Check sheet for the drawn part. Datum: minimum x, y, z corner. Units: mm. A direction names the side the tool comes from. Give positions to 0.01 mm unless a question says otherwise; leave off trailing zeros. Loops run counter-clockwise (first coordinate to the right, second up) from the corner with the lowest first, then second, coordinate; pieces in that order, holes last. Notation, with made-up numbers: (33.5, 71.5) - (59.5, 71.5) arc R22 ccw to (59.5, 106.5) - close; hole circle Ø2 at (23, 10.25). An arc over 180 degrees is marked (long way). Use one line per item in the form item = value.
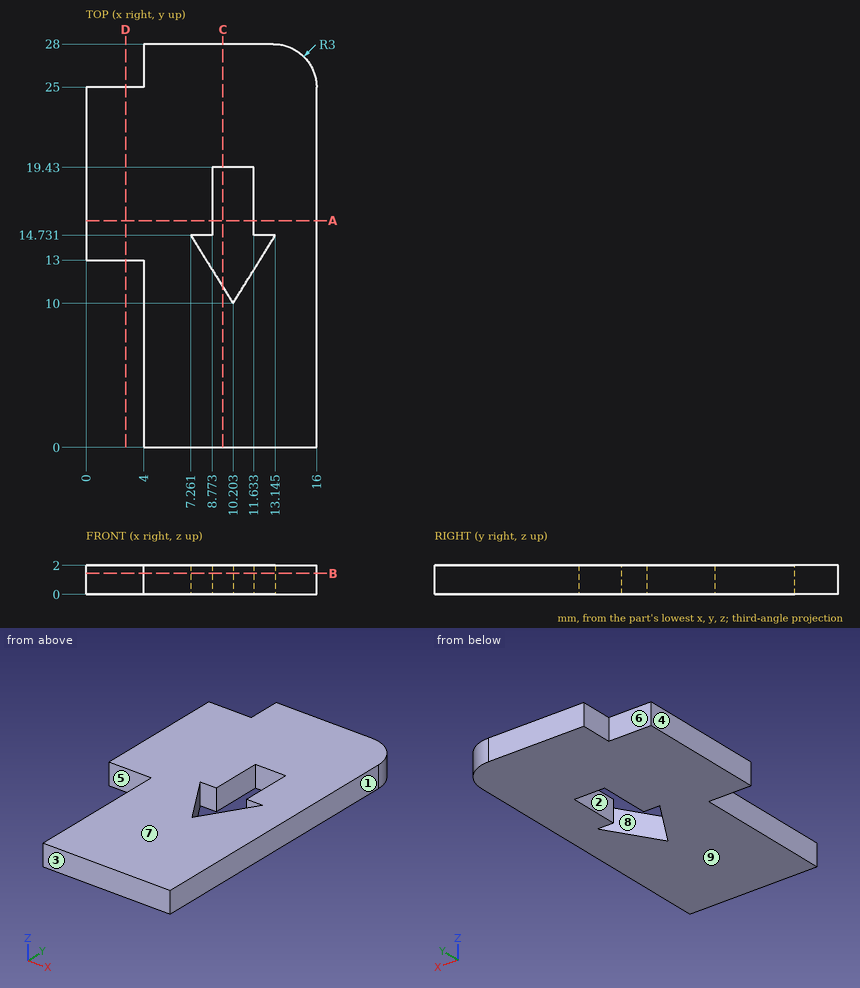
Item 1: Section check A-A on y = 15.75. Record the boundary of the cut face in (x, z), then the cut area to 3 significant figures.
Answer block:
outline = (0, 0) - (8.77, 0) - (8.77, 2) - (0, 2) - close; (11.63, 0) - (16, 0) - (16, 2) - (11.63, 2) - close
area = 26.3 mm2
Item 2: Gauge pin test, flat ends, axial feed: P1, Ø1, axis at y = 12, z = 1.5, coming from the -X side; P2, Ø0.6, axis at x = 1, z = 1, coming from the -Y side. Record the tip position at first contact, or that the pin passes through.
Answer block:
P1 = 4
P2 = 13
Item 3: Section check B-B on z = 1.45. Record the boundary of the cut face in (x, y) (1 decimal), then the cut area to 3 significant figures.
Answer block:
outline = (0, 13) - (4, 13) - (4, 0) - (16, 0) - (16, 25) arc R3 ccw to (13, 28) - (4, 28) - (4, 25) - (0, 25) - close; hole (7.3, 14.7) - (10.2, 10) - (13.1, 14.7) - (11.6, 14.7) - (11.6, 19.4) - (8.8, 19.4) - (8.8, 14.7) - close
area = 355 mm2
Item 4: Thickness scan on L1, parallel to X at y = 4, z = 0.75; L2, parallel to Y at x = 2.75, z = 0.5; L3, parallel to X at y = 12.75, z = 0.95. Record the ranges inside material, lowest first.
Answer block:
L1 = 4 to 16
L2 = 13 to 25
L3 = 4 to 8.49, 11.91 to 16
Item 5: Mould release check, pull along X, two halves, no side actions. Record for the marked faces 1, 2, 3 and 4: released by +X, released by -X, zero draft, split by the parting line, or undercut.
Answer block:
face_1 = released by +X
face_2 = undercut
face_3 = zero draft
face_4 = released by -X
Item 6: Section check C-C on x = 9.5. Record the boundary of the cut face in (y, z).
Answer block:
outline = (0, 0) - (11.13, 0) - (11.13, 2) - (0, 2) - close; (19.43, 0) - (28, 0) - (28, 2) - (19.43, 2) - close
Item 7: Section check D-D on x = 2.75. Record the boundary of the cut face in (y, z).
Answer block:
outline = (13, 0) - (25, 0) - (25, 2) - (13, 2) - close
Item 8: Access from +Z, -Z, +X, -X, +Y, -Y to the whole of each face (thin tool, end or side, straight path). Record for the marked faces 5, 6, 7, 8 and 9.
Answer block:
face_5 = +Z, -Z, -X, -Y
face_6 = +Z, -Z, -X, +Y
face_7 = +Z, +X, -X, +Y, -Y
face_8 = +Z, -Z
face_9 = -Z, +X, -X, +Y, -Y
